Verification items for the finished model (mm, model axes). Coordinates: 2 decimals unless noted, no trailing zeros. Loops run counter-clockwise (first coordinate to the right, second up) from the corner with the lowest first, then second, coordinate; pieces in that order, holes last. Notation, with made-up numbers: M -2,5 L 21,5 A20 cw 21,23 Z; hole C 65.5,-15.5 d4. An arc over 180 degrees is marked long. Write item = value, one per line. Start each with the question number.
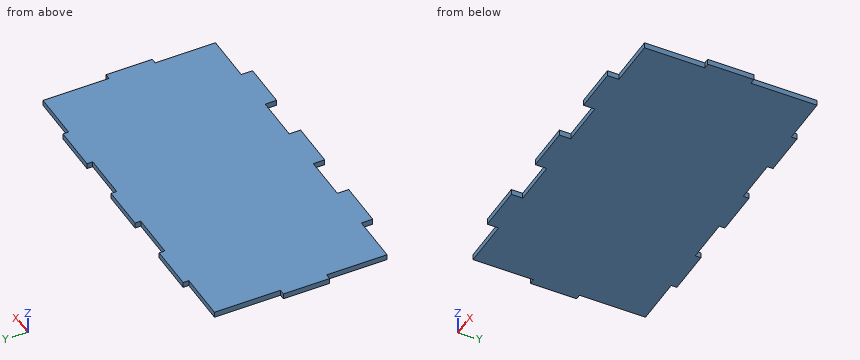
```python
from build123d import *

# Parameters (mm, degrees)
SALIENTE_EXTRUIR1_DEPTH = 3
CROQUIS1_W              = 26.025
CROQUIS1_H              = 3
CROQUIS1_W_2            = 24.39
CORTAR_EXTRUIR1_DEPTH   = 3


with BuildPart() as part:
    # Model → Saliente-Extruir1 (new body)
    with BuildSketch(Plane.XY):
        Polygon((289, 97), (289, 62.195), (286, 62.195), (286, 37.805), (289, 37.805), (289, 13.415), (289, 3), (315.025, 3), (315.025, 0), (339.415, 0), (339.415, 3), (363.805, 3), (363.805, 0), (388.195, 0), (388.195, 3), (412.585, 3), (412.585, 0), (436.975, 0), (436.975, 3), (461.365, 3), (463, 3), (463, 37.805), (466, 37.805), (466, 62.195), (463, 62.195), (463, 86.585), (463, 97), (436.975, 97), (436.975, 100), (412.585, 100), (412.585, 97), (388.195, 97), (388.195, 100), (363.805, 100), (363.805, 97), (339.415, 97), (339.415, 100), (315.025, 100), (315.025, 97), (290.635, 97), align=None)
    extrude(amount=SALIENTE_EXTRUIR1_DEPTH)

    # Croquis1 → Cortar-Extruir1 (cut)
    with BuildSketch(Plane.XY.offset(3)):
        with Locations((302.0125, 4.5)):
            Rectangle(CROQUIS1_W, CROQUIS1_H)
        with Locations((351.61, 4.5)):
            Rectangle(CROQUIS1_W_2, CROQUIS1_H)
        with Locations((400.39, 4.5)):
            Rectangle(CROQUIS1_W_2, CROQUIS1_H)
        with Locations((449.9875, 4.5)):
            Rectangle(CROQUIS1_W, CROQUIS1_H)
    extrude(amount=-CORTAR_EXTRUIR1_DEPTH, mode=Mode.SUBTRACT)


solid = part.part
```
Q1. Sectioned sample at A-A on y = 65. Record the cut outline in (x, z), plus the area to 3 significant figures.
Q2. Gauge pin test, flat ends, axial feed: pin 1 (1.5 mm diameter, centred on y = 4, z = 1, fed in from +X) (3 decimals); pin 2 (1.5 mm diameter, centred on y = 98.5, z = 1.5, fed in from -X) (3 decimals); pin 3 (1.5 mm diameter, centred on x = 447, z = 1, fed in from +Y). Record the tip position at first contact, or that the pin passes through.
Q3. Sectioned sample at B-B on x = 358.5. Record the cut outline in (y, z), plus the area to 3 significant figures.
Q4. Scan lines: L1, parallel to X at y = 94.5, z = 0.8; L2, parallel to Y at x = 353, z = 0.8. Record each from-to range of solid material in increasing order. Write a range as [from, to].
Solutions:
q1.outline = M 289,0 L 463,0 L 463,3 L 289,3 Z
q1.area = 522 mm²
q2.pin_1 = 436.975
q2.pin_2 = 315.025
q2.pin_3 = 97
q3.outline = M 6,0 L 97,0 L 97,3 L 6,3 Z
q3.area = 273 mm²
q4.L1 = [289, 463]
q4.L2 = [6, 97]
